```python
from build123d import *

# Parameters (mm, degrees)
BOX004_W                  = 4
BOX004_H                  = 10
BOX004_DEPTH              = 10
CYLINDER002_R             = 5
CYLINDER002_DEPTH         = 10
BOX003_W                  = 4
BOX003_H                  = 10
BOX003_DEPTH              = 10
CYLINDER001_R             = 5
CYLINDER001_DEPTH         = 10
BOX001_W                  = 15
BOX001_H                  = 10
BOX001_DEPTH              = 8
FILLET002_R               = 3
LID_GROOVE_LEFT_R         = 1.1
LID_GROOVE_LEFT_DEPTH     = 66.8
LID_GROOVE_RIGHT_R        = 1.1
LID_GROOVE_RIGHT_DEPTH    = 66.8
LID_INSIDE_W              = 325.8
LID_INSIDE_H              = 85.8
LID_INSIDE_DEPTH          = 4
LID_OUTSIDE_W             = 330
LID_OUTSIDE_H             = 90
LID_OUTSIDE_DEPTH         = 6.1
FILLET001_R               = 1
FILLET001_PLACEMENT_ANGLE = 180


with BuildPart() as cube003:
    # Box004 → Box004 (new body)
    with BuildSketch(Plane.XY):
        with Locations((2, 5)):
            Rectangle(BOX004_W, BOX004_H)
    extrude(amount=BOX004_DEPTH)


with BuildPart() as fusion002:
    # Cylinder002 → Cylinder002 (new body)
    with BuildSketch(Plane(origin=(2, 13, 0), x_dir=(1, 0, 0), z_dir=(0, 0, 1))):
        Circle(CYLINDER002_R)
    extrude(amount=CYLINDER002_DEPTH)

    # Fusion002: union Cube003
    add(cube003.part)


with BuildPart() as fusion002_1:
    # Fusion002 placement: moved
    add(fusion002.part.moved(Location((258.5, 25, 8))))


with BuildPart() as cube002:
    # Box003 → Box003 (new body)
    with BuildSketch(Plane.XY):
        with Locations((2, 5)):
            Rectangle(BOX003_W, BOX003_H)
    extrude(amount=BOX003_DEPTH)


with BuildPart() as fusion001:
    # Cylinder001 → Cylinder001 (new body)
    with BuildSketch(Plane(origin=(2, 13, 0), x_dir=(1, 0, 0), z_dir=(0, 0, 1))):
        Circle(CYLINDER001_R)
    extrude(amount=CYLINDER001_DEPTH)

    # Fusion001: union Cube002
    add(cube002.part)


with BuildPart() as fusion001_1:
    # Fusion001 placement: moved
    add(fusion001.part.moved(Location((58.5, 25, 8))))


with BuildPart() as fillet002:
    # Box001 → Box001 (new body)
    with BuildSketch(Plane(origin=(153.5, 80, 2), x_dir=(1, 0, 0), z_dir=(0, 0, 1))):
        with Locations((7.5, 5)):
            Rectangle(BOX001_W, BOX001_H)
    extrude(amount=BOX001_DEPTH)

    # Fillet002
    fillet002_edges = [fillet002.edges().sort_by_distance(p)[0] for p in [
        (153.5, 85, 10),
        (153.5, 85, 2),
        (168.5, 85, 10),
        (168.5, 85, 2),
    ]]
    fillet(fillet002_edges, radius=FILLET002_R)


with BuildPart() as lid_groove_left:
    # lid_groove_left → lid_groove_left (new body)
    with BuildSketch(Plane(origin=(-2.4, 7.1, 1), x_dir=(1, 0, 0), z_dir=(0, 1, 0))):
        Circle(LID_GROOVE_LEFT_R)
    extrude(amount=LID_GROOVE_LEFT_DEPTH)


with BuildPart() as lid_groove_right:
    # lid_groove_right → lid_groove_right (new body)
    with BuildSketch(Plane(origin=(323.4, 7.1, 1), x_dir=(1, 0, 0), z_dir=(0, 1, 0))):
        Circle(LID_GROOVE_RIGHT_R)
    extrude(amount=LID_GROOVE_RIGHT_DEPTH)


with BuildPart() as lid_inside:
    # lid_inside → lid_inside (new body)
    with BuildSketch(Plane(origin=(-2.4, -2.4, 0), x_dir=(1, 0, 0), z_dir=(0, 0, 1))):
        with Locations((162.9, 42.9)):
            Rectangle(LID_INSIDE_W, LID_INSIDE_H)
    extrude(amount=LID_INSIDE_DEPTH)


with BuildPart() as lid002:
    # lid_outside → lid_outside (new body)
    with BuildSketch(Plane(origin=(-4.5, -4.5, -2.1), x_dir=(1, 0, 0), z_dir=(0, 0, 1))):
        with Locations((165, 45)):
            Rectangle(LID_OUTSIDE_W, LID_OUTSIDE_H)
    extrude(amount=LID_OUTSIDE_DEPTH)

    # Cut001: cut lid_inside
    add(lid_inside.part, mode=Mode.SUBTRACT)

    # Cut002: cut lid_groove_right
    add(lid_groove_right.part, mode=Mode.SUBTRACT)

    # Cut003: cut lid_groove_left
    add(lid_groove_left.part, mode=Mode.SUBTRACT)

    # Fillet001
    fillet001_edges = [lid002.edges().sort_by_distance(p)[0] for p in [
        (-4.5, -4.5, 0.95),
        (-4.5, 85.5, 0.95),
        (-4.5, 40.5, -2.1),
        (160.5, -4.5, -2.1),
        (325.5, -4.5, 0.95),
        (160.5, 85.5, -2.1),
        (325.5, 85.5, 0.95),
        (325.5, 40.5, -2.1),
    ]]
    fillet(fillet001_edges, radius=FILLET001_R)


with BuildPart() as lid002_1:
    # Fillet001 placement: moved
    add(lid002.part.moved(Location((0, 81, 10))).rotate(Axis((0, 81, 10), (1, 0, 0)), FILLET001_PLACEMENT_ANGLE))

    # Cut004: cut Fillet002
    add(fillet002.part, mode=Mode.SUBTRACT)

    # Cut007: cut Fusion001
    add(fusion001_1.part, mode=Mode.SUBTRACT)

    # Cut008: cut Fusion002
    add(fusion002_1.part, mode=Mode.SUBTRACT)


solid = lid002_1.part
```
For this review, take the finished solid that the model builds, in its own axes (mm). Coordinates: 2 decimals unless noted, no trailing zeros. Loops run counter-clockwise (first coordinate to the right, second up) from the corner with the lowest first, then second, coordinate; pieces in that order, holes last.
1. Insertion check: P1, Ø8, axis at x = 186, y = 19, coming from the -Z side. The pin has a flat end and moves straight along its axis. Give the tip position at first contact, or say it passes through.
2. Add section A-A, the plane y = 13. Give the boundary of the cut face in (x, z).
3. Add section C-C, the plane z = 9. Give the boundary of the cut face in (x, y), then the cut area to 3 significant figures.
4. For line 1 (X direction, y = 38, z = 11.4); line 2 (Y direction, x = 56, z = 9.25); line 3 (X direction, y = 31, z = 8.75), list the stretches that pass through material, from the lowest coordinate up.
5. Mouldability with a two-part tool opening along Y and no side actions: class faces 1 (the flat face through (158, 40, 12.1)), 2 (the cylindrical face through (60.691, 42.996, 11.035)), 3 (the flat face through (158, 42, 10)) as +Y half, -Y half, draft (parallel to the pull), parting line (faces both ways), or undercut.
6. Add section B-B, the plane x = 144. Give the boundary of the cut face in (y, z), then the cut area to 3 significant figures.
Result:
1. P1: stops at z = 10
2. outline: (-4.5, 6) - (-2.4, 6) - (-2.4, 7.9) arc R1.1 cw (long way) to (-1.94, 10) - (322.94, 10) arc R1.1 cw (long way) to (323.4, 7.9) - (323.4, 6) - (325.5, 6) - (325.5, 11.1) arc R1 ccw to (324.5, 12.1) - (-3.5, 12.1) arc R1 ccw to (-4.5, 11.1) - close
3. outline: (-4.5, -3.5) arc R1 ccw to (-3.5, -4.5) - (324.5, -4.5) arc R1 ccw to (325.5, -3.5) - (325.5, 84.5) arc R1 ccw to (324.5, 85.5) - (167.74, 85.5) - (167.74, 83.4) - (323.4, 83.4) - (323.4, 73.9) - (324.5, 73.9) - (324.5, 7.1) - (323.4, 7.1) - (323.4, -2.4) - (-2.4, -2.4) - (-2.4, 7.1) - (-3.5, 7.1) - (-3.5, 73.9) - (-2.4, 73.9) - (-2.4, 83.4) - (154.26, 83.4) - (154.26, 85.5) - (-3.5, 85.5) arc R1 ccw to (-4.5, 84.5) - close
3. area: 1,570 mm2
4. line 1: x = -4.45 to 55.5, 65.5 to 255.5, 265.5 to 325.45
4. line 2: y = -4.5 to -2.4, 83.4 to 85.5
4. line 3: x = -4.5 to -3.47, 324.47 to 325.5
5. face 1: draft
5. face 2: undercut
5. face 3: undercut
6. outline: (-4.5, 6) - (-2.4, 6) - (-2.4, 10) - (83.4, 10) - (83.4, 6) - (85.5, 6) - (85.5, 11.1) arc R1 ccw to (84.5, 12.1) - (-3.5, 12.1) arc R1 ccw to (-4.5, 11.1) - close
6. area: 205 mm2
